```python
from build123d import *

# Parameters (mm, degrees)
F0_R     = 88.9
F0_R_2   = 12.7
F0_R_3   = 34.925
F1_DEPTH = 6.35
F0_R_4   = 25.4
F2_DEPTH = 12.7


with BuildPart() as f1:
    # F0 (on Front) → F1 (new body)
    with BuildSketch(Plane.XZ):
        Circle(F0_R)
        with Locations((-54.992613, -31.75)):
            Circle(F0_R_2, mode=Mode.SUBTRACT)
        with Locations((54.992613, -31.75)):
            Circle(F0_R_2, mode=Mode.SUBTRACT)
        Circle(F0_R_3, mode=Mode.SUBTRACT)
        with Locations((0, 63.5)):
            Circle(F0_R_2, mode=Mode.SUBTRACT)
    extrude(amount=F1_DEPTH)

    # F0 (on Front) → F2 (join)
    with BuildSketch(Plane.XZ):
        Circle(F0_R_3)
        Circle(F0_R_4, mode=Mode.SUBTRACT)
    extrude(amount=F2_DEPTH)


solid = f1.part
```
Build history of the part. All positions in model axes, mm. A direction names the side the tool comes from. Give positions to 0.01 mm unless a question says otherwise; leave off trailing zeros. Loops run counter-clockwise (first coordinate to the right, second up) from the corner with the lowest first, then second, coordinate; pieces in that order, holes last. Notation, with made-up numbers: (67, 3.5) - (119, 3.5) arc R13 cw to (119, 21.5) - close; hole circle Ø3 at (41, 14.25). An arc over 180 degrees is marked (long way). Use a Markdown table: item, result.
(1) Band-saw the part on D-D (x = 62.5). Give the cut face in (y, z).
Taken from the geometry:
| item | result |
|---|---|
| outline | (-6.35, -63.22) - (0, -63.22) - (0, -41.99) - (-6.35, -41.99) - close; (-6.35, -21.51) - (0, -21.51) - (0, 63.22) - (-6.35, 63.22) - close |
(2) Wall check: line 1 along Z through (x, y) = (0, -1.75); line 2 along X through (y, z) = (-1.25, -20.5); line 3 along Y through (x, z) = (-78, 14). Give the ranges that are in metal, low to high.
Taken from the geometry:
| item | result |
|---|---|
| line 1 | -88.9 to -25.4, 25.4 to 50.8, 76.2 to 88.9 |
| line 2 | -86.5 to -60.89, -49.1 to -15, 15 to 49.1, 60.89 to 86.5 |
| line 3 | -6.35 to 0 |
(3) Drop flat-ended pins along their axis: pin 1 Ø4 at (x, z) = (65, 13) entering from -Y; pin 2 Ø20.5 at (x, z) = (-54.99, -31.75) entering from +Y; pin 3 Ø1.5 at (x, y) = (-14.5, -7) entering from -Z; pin 4 Ø3 at (y, z) = (-11, 27.5) entering from +X. Give the stop position or say it passes through.
Taken from the geometry:
| item | result |
|---|---|
| pin 1 | y = -6.35 |
| pin 2 | through |
| pin 3 | z = -87.77 |
| pin 4 | x = 23.32 |
(4) Pull direction X, two halves, no side cores. Call faces 1 (the face through (66.724, -3.131, -36.614)), 2 (the face through (-27.715, -9.481, -21.251)), 3 (the face through (19, 0, -19)): +X half, -X half, draft (parallel to the pull), parting line (faces both ways), or undercut.
Taken from the geometry:
| item | result |
|---|---|
| face 1 | undercut |
| face 2 | parting line |
| face 3 | draft |
(5) Band-saw the part on C-C (y = -4). Give the cut face in (x, z), and give its area (3 significant figures).
Taken from the geometry:
| item | result |
|---|---|
| outline | circle Ø177.8 at (0, 0); hole circle Ø25.4 at (-54.99, -31.75); hole circle Ø50.8 at (0, 0); hole circle Ø25.4 at (0, 63.5); hole circle Ø25.4 at (54.99, -31.75) |
| area | 21,300 mm2 |
(6) Band-saw the part on B-B (x = 4). Give the cut face in (y, z), and give its area (3 significant figures).
Taken from the geometry:
| item | result |
|---|---|
| outline | (-12.7, -34.7) - (-6.35, -34.7) - (-6.35, -88.81) - (0, -88.81) - (0, -25.08) - (-12.7, -25.08) - close; (-12.7, 25.08) - (0, 25.08) - (0, 51.45) - (-6.35, 51.45) - (-6.35, 34.7) - (-12.7, 34.7) - close; (-6.35, 75.55) - (0, 75.55) - (0, 88.81) - (-6.35, 88.81) - close |
| area | 778 mm2 |
(7) Which spindle directions (+Z, -Z, +X, -X, +Y, -Y) get a long thin tool onto all of the face, cutting with end or side? Do faces 4 (the face through (38, -6.35, 1)), 5 (the face through (2, -12.7, -26)). Say none if no direction does.
Taken from the geometry:
| item | result |
|---|---|
| face 4 | -Y |
| face 5 | +Z, -Z, +X, -X, -Y |
(8) Band-saw the part on A-A (z = 0). Give the cut face in (x, y) (3 decimals), and give its area (3 significant figures).
Taken from the geometry:
| item | result |
|---|---|
| outline | (-88.9, -6.35) - (-34.925, -6.35) - (-34.925, -12.7) - (-25.4, -12.7) - (-25.4, 0) - (-88.9, 0) - close; (25.4, -12.7) - (34.925, -12.7) - (34.925, -6.35) - (88.9, -6.35) - (88.9, 0) - (25.4, 0) - close |
| area | 927 mm2 |
